Verification items for the finished model (mm, model axes). A direction names the side the tool comes from. Round coordinates to 2 decimals unless told otherwise and drop trailing zeros. Write each loop counter-clockwise with the first axis right and the second up, starting at its lowest first coordinate (ties: lowest second). Pieces come first, ordered by that corner, then holes. Notation, with made-up numbers: M -15.75,-6 L -4.75,-6 A25 cw -4.75,24 Z; hole C -26,19.5 d10. An arc over 180 degrees is marked long. One line per item, written item: value. Start each with the question number.
Item 1: Gauge pin test, flat end, axial feed: pin 1 (3 mm diameter, centred on x = -0.5, y = 0.5, fed in from +Z). Record the tip position at first contact, or that the pin passes through.
Item 2: Section check C-C, the plane z = 2.5. Record the cut outline in (x, y).
Item 3: Section check A-A, the plane y = -0.4. Record the cut outline in (x, z).
Item 4: Thickness scan on probe 1 along X at (y, z) = (-0.3, 0.75); probe 2 along Y at (x, z) = (-2, 1.75); probe 3 along Z at (x, y) = (11, -1.7). Record the ranges inside material, lowest first. Write a range as from..to.
Item 5: Section check B-B, the plane x = 13. Record the cut outline in (y, z).
Item 6: Draft check along X on faces 3 (the face through (-18.4, 0, 4)), 4 (the face through (0, 1.4, 4)), 5 (the face through (0, -2.9, 4)). Enter one of: +X half, -X half, draft (parallel to the pull), parting line (faces both ways), or undercut.
Item 7: Tool access check on faces 1 (the face through (-16.9, 0, 4)), 2 (the face through (0, 2.9, 4)). Record the directions out of +Z, -Z, +X, -X, +Y, -Y that give a thin tool (end or side, any length) a straight path to the whole face; none if there is none.
from build123d import *

# Parameters (mm, degrees)
SKETCH_W     = 36.8
SKETCH_H     = 5.8
SKETCH_W_2   = 33.8
SKETCH_H_2   = 2.8
PAD_DEPTH    = 9
CHAMFER_SIZE = 0.75


with BuildPart() as part:
    # Sketch → Pad (new body)
    with BuildSketch(Plane.XY):
        Rectangle(SKETCH_W, SKETCH_H)
        Rectangle(SKETCH_W_2, SKETCH_H_2, mode=Mode.SUBTRACT)
    extrude(amount=PAD_DEPTH)

    # Chamfer
    chamfer_edges = [part.edges().sort_by_distance(p)[0] for p in [
        (0, 1.4, 9),
        (0, -1.4, 9),
        (-16.9, 0, 9),
        (16.9, 0, 9),
    ]]
    chamfer(chamfer_edges, length=CHAMFER_SIZE)


solid = part.part
Response values:
1. pin 1: stops at z = 8.85
2. outline: M -18.4,-2.9 L 18.4,-2.9 L 18.4,2.9 L -18.4,2.9 Z; hole M -16.9,-1.4 L 16.9,-1.4 L 16.9,1.4 L -16.9,1.4 Z
3. outline: M -18.4,0 L -16.9,0 L -16.9,8.25 L -17.65,9 L -18.4,9 Z; M 16.9,0 L 18.4,0 L 18.4,9 L 17.65,9 L 16.9,8.25 Z
4. probe 1: x = -18.4..-16.9, 16.9..18.4
4. probe 2: y = -2.9..-1.4, 1.4..2.9
4. probe 3: z = 0..8.55
5. outline: M -2.9,0 L -1.4,0 L -1.4,8.25 L -2.15,9 L -2.9,9 Z; M 1.4,0 L 2.9,0 L 2.9,9 L 2.15,9 L 1.4,8.25 Z
6. face 3: -X half
6. face 4: undercut
6. face 5: draft
7. face 1: +Z, -Z
7. face 2: +Z, -Z, +X, -X, +Y
